Design review of the part built by this model. Coordinates are the model's own, in mm. Face numbers are marked on the shaded views. A direction names the side the tool comes from. Give positions to 0.01 mm unless a question says otherwise; leave off trailing zeros. Order: outer loops, then holes, each group sorted by start corner. A loop starts at its lowest first (then second) coordinate and runs counter-clockwise, first axis right, second up. Notation, with made-up numbers: (63.5, 28) -> (88.5, 28) arc R25 cw to (88.5, 55) -> close; hole circle Ø10 at (42.5, 28). An arc over 180 degrees is marked (long way). Answer in a Markdown table with one row per item. Add a question column.
```python
from build123d import *

# Parameters (mm, degrees)
BOSS_EXTRUDE1_DEPTH = 7.5
CUT_EXTRUDE1_REACH  = 57
SKETCH2_R           = 1.65


with BuildPart() as part:
    # Sketch1 → Boss-Extrude1 (new body, symmetric)
    with BuildSketch(Plane.XY):
        Polygon((-37.5, 0), (37.5, 0), (37.5, -40), (47.5, -40), (47.5, 10), (-47.5, 10), (-47.5, -45), (-37.5, -45), align=None)
    extrude(amount=BOSS_EXTRUDE1_DEPTH, both=True)

    # Sketch2 → Cut-Extrude1 (cut, up to next)
    with BuildSketch(Plane(origin=(0, 10, 0), x_dir=(1, 0, 0), z_dir=(0, 1, 0)), mode=Mode.PRIVATE) as cut_extrude1_sk1:
        with Locations((-10, 0)):
            Circle(SKETCH2_R)
    cut_extrude1_tool1 = extrude(cut_extrude1_sk1.sketch, amount=-CUT_EXTRUDE1_REACH, mode=Mode.PRIVATE) & part.part
    add(cut_extrude1_tool1.solids().sort_by_distance((-10, 10, 0))[0], mode=Mode.SUBTRACT)
    # Sketch2 → Cut-Extrude1 (cut, up to next)
    with BuildSketch(Plane(origin=(0, 10, 0), x_dir=(1, 0, 0), z_dir=(0, 1, 0)), mode=Mode.PRIVATE) as cut_extrude1_sk2:
        with Locations((10, 0)):
            Circle(SKETCH2_R)
    cut_extrude1_tool2 = extrude(cut_extrude1_sk2.sketch, amount=-CUT_EXTRUDE1_REACH, mode=Mode.PRIVATE) & part.part
    add(cut_extrude1_tool2.solids().sort_by_distance((10, 10, 0))[0], mode=Mode.SUBTRACT)
    # Sketch2 → Cut-Extrude1 (cut, up to next)
    with BuildSketch(Plane(origin=(0, 10, 0), x_dir=(1, 0, 0), z_dir=(0, 1, 0)), mode=Mode.PRIVATE) as cut_extrude1_sk3:
        with Locations((20, 0)):
            Circle(SKETCH2_R)
    cut_extrude1_tool3 = extrude(cut_extrude1_sk3.sketch, amount=-CUT_EXTRUDE1_REACH, mode=Mode.PRIVATE) & part.part
    add(cut_extrude1_tool3.solids().sort_by_distance((20, 10, 0))[0], mode=Mode.SUBTRACT)
    # Sketch2 → Cut-Extrude1 (cut, up to next)
    with BuildSketch(Plane(origin=(0, 10, 0), x_dir=(1, 0, 0), z_dir=(0, 1, 0)), mode=Mode.PRIVATE) as cut_extrude1_sk4:
        with Locations((-20, 0)):
            Circle(SKETCH2_R)
    cut_extrude1_tool4 = extrude(cut_extrude1_sk4.sketch, amount=-CUT_EXTRUDE1_REACH, mode=Mode.PRIVATE) & part.part
    add(cut_extrude1_tool4.solids().sort_by_distance((-20, 10, 0))[0], mode=Mode.SUBTRACT)


solid = part.part
```
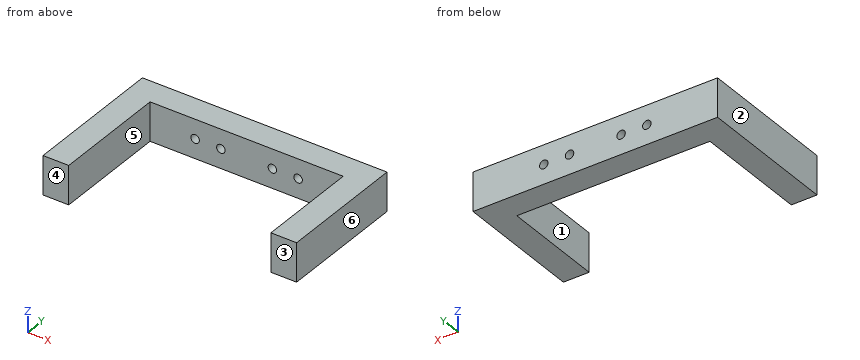
1) Add section C-C, the plane y = -23. Write out the cut boundary in (x, z), and give its area (3 significant figures).
2) Mouldability with a two-part tool opening along X and no side actions: class the marked faces 4, 5 and 6 as +X half, -X half, draft (parallel to the pull), parting line (faces both ways), or undercut.
3) For L1, parallel to X at y = 2.75, z = 0; L2, parallel to X at y = -33.5, z = 4; L3, parallel to Z at x = 20, y = 6.75, list the stretches that pass through material, from the lowest coordinate up.
4) Machinability: for the marked faces 1, 2 and 3, which of the approach directions +Z, -Z, +X, -X, +Y, -Y give a long, thin tool a straight path to every point of the face, cutting with its end or side? Answer none if there is none.
5) Add section B-B, the plane z = 0. Write out the cut boundary in (x, y), and give its area (3 significant figures).
6) Add section A-A, the plane x = -20. Write out the cut boundary in (y, z), and give its area (3 significant figures).
7) Clearance check with flat-ended pins moving along their axes: P1, Ø8, axis at x = 34, z = -3.5, coming from the -Y side; P2, Ø5, axis at x = -16.5, z = -2, coming from the -Y side. State where each tip first meets the part, or that it passes through.
8) Add section D-D, the plane z = -5. Write out the cut boundary in (x, y).
Verdict:
| question | item | result |
|---|---|---|
| 1 | outline | (-47.5, -7.5) -> (-37.5, -7.5) -> (-37.5, 7.5) -> (-47.5, 7.5) -> close; (37.5, -7.5) -> (47.5, -7.5) -> (47.5, 7.5) -> (37.5, 7.5) -> close |
| 1 | area | 300 mm2 |
| 2 | face 4 | draft |
| 2 | face 5 | undercut |
| 2 | face 6 | +X half |
| 3 | L1 | x = -47.5 to -21.65, -18.35 to -11.65, -8.35 to 8.35, 11.65 to 18.35, 21.65 to 47.5 |
| 3 | L2 | x = -47.5 to -37.5, 37.5 to 47.5 |
| 3 | L3 | z = -7.5 to -1.65, 1.65 to 7.5 |
| 4 | face 1 | +Z, -Z, -Y |
| 4 | face 2 | +Z, -Z, -X, +Y, -Y |
| 4 | face 3 | +Z, -Z, +X, -Y |
| 5 | outline | (-47.5, -45) -> (-37.5, -45) -> (-37.5, 0) -> (-21.65, 0) -> (-21.65, 10) -> (-47.5, 10) -> close; (-18.35, 0) -> (-11.65, 0) -> (-11.65, 10) -> (-18.35, 10) -> close; (-8.35, 0) -> (8.35, 0) -> (8.35, 10) -> (-8.35, 10) -> close; (11.65, 0) -> (18.35, 0) -> (18.35, 10) -> (11.65, 10) -> close; (21.65, 0) -> (37.5, 0) -> (37.5, -40) -> (47.5, -40) -> (47.5, 10) -> (21.65, 10) -> close |
| 5 | area | 1,670 mm2 |
| 6 | outline | (0, -7.5) -> (10, -7.5) -> (10, -1.65) -> (0, -1.65) -> close; (0, 1.65) -> (10, 1.65) -> (10, 7.5) -> (0, 7.5) -> close |
| 6 | area | 117 mm2 |
| 7 | P1 | stops at y = -40 |
| 7 | P2 | stops at y = 0 |
| 8 | outline | (-47.5, -45) -> (-37.5, -45) -> (-37.5, 0) -> (37.5, 0) -> (37.5, -40) -> (47.5, -40) -> (47.5, 10) -> (-47.5, 10) -> close |
